Design review of the part built by this model. Coordinates are the model's own, in mm. Face numbers are marked on the shaded views. Coordinates: 2 decimals unless noted, no trailing zeros. Order: outer loops, then holes, each group sorted by start corner. A loop starts at its lowest first (then second) coordinate and runs counter-clockwise, first axis right, second up. Notation, with made-up numbers: (-37, 31.5) -> (6, 31.5) arc R24 ccw to (6, 50.5) -> close; hole circle Ø6 at (69.5, -5.75). An arc over 180 degrees is marked (long way). Use a Markdown table: item, result. Add a question column.
Q1. Add section C-C (y = 41). State the section outline as (x, z) points.
Q2. Add section D-D (x = 0). State the section outline as (y, z) points, then the cut area to 3 significant figures.
Q3. The part is to be moulded in two halves that separate along X. For the marked faces 1 and 2, say which applies: pulls with the +X half, pulls with the -X half, needs draft (parallel to the pull), parting line crosses it, or undercut.
Q4. Insertion check: pin 1 (0.5 mm diameter, centred on x = 1, z = 0, fed in from -Y); pin 2 (2 mm diameter, centred on x = -0.5, y = 3.5, fed in from +Z); pin 3 (2 mm diameter, centred on y = 7.5, z = -1.5, fed in from +X). Each pin has a flat end and moves straight along its axis. Give the tip position at first contact, or say it passes through.
Q5. Add section B-B (z = 0). State the section outline as (x, y) points.
Q6. Add section A-A (x = -2.2). State the section outline as (y, z) points.
Q7. Wall thickness on probe 1 along Y at (x, z) = (1.1, -1.85); probe 2 along Y at (x, z) = (-0.2, 0.3); probe 3 along Z at (x, y) = (1.05, 1): over which ranges is each line inside the solid? List them lowest first.
from build123d import *

# Parameters (mm, degrees)
F0_R     = 2.75
F1_DEPTH = 2
F3_DEPTH = 0.7
F4_R     = 1.5
F5_DEPTH = 45


with BuildPart() as f1:
    # F0 (on Front) → F1 (new body)
    with BuildSketch(Plane.XZ):
        Circle(F0_R)
    extrude(amount=F1_DEPTH)

    # F2 (on face) → F3 (cut)
    with BuildSketch(Plane.XZ.offset(2)):
        with BuildLine():
            ThreePointArc((2.75, 0), (2.7385168893, 0.2510482965), (2.7041634566, 0.5))
            Line((2.7041634566, 0.5), (-2.7041634566, 0.5))
            ThreePointArc((-2.7041634566, 0.5), (-2.75, 0), (-2.7041634566, -0.5))
            Line((-2.7041634566, -0.5), (2.7041634566, -0.5))
            ThreePointArc((2.7041634566, -0.5), (2.7385168893, -0.2510482965), (2.75, 0))
        make_face()
    extrude(amount=-F3_DEPTH, mode=Mode.SUBTRACT)

    # F4 (on face) → F5 (join)
    with BuildSketch(Plane(origin=(0, 0, 0), x_dir=(-1, 0, 0), z_dir=(0, 1, 0))):
        Circle(F4_R)
    extrude(amount=F5_DEPTH)


solid = f1.part
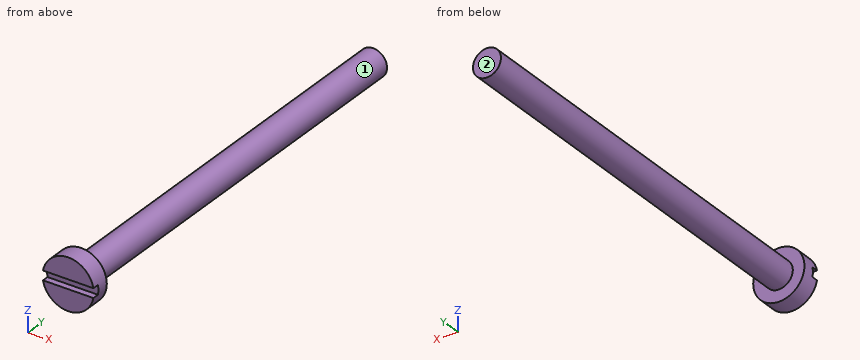
Established:
| question | item | result |
|---|---|---|
| 1 | outline | circle Ø3 at (0, 0) |
| 2 | outline | (-2, -2.75) -> (0, -2.75) -> (0, -1.5) -> (45, -1.5) -> (45, 1.5) -> (0, 1.5) -> (0, 2.75) -> (-2, 2.75) -> (-2, 0.5) -> (-1.3, 0.5) -> (-1.3, -0.5) -> (-2, -0.5) -> close |
| 2 | area | 145 mm^2 |
| 3 | face 1 | parting line crosses it |
| 3 | face 2 | needs draft |
| 4 | pin 1 | y = -1.3 |
| 4 | pin 2 | z = 1.5 |
| 4 | pin 3 | x = 1.41 |
| 5 | outline | (-2.75, -1.3) -> (2.75, -1.3) -> (2.75, 0) -> (1.5, 0) -> (1.5, 45) -> (-1.5, 45) -> (-1.5, 0) -> (-2.75, 0) -> close |
| 6 | outline | (-2, -1.65) -> (0, -1.65) -> (0, 1.65) -> (-2, 1.65) -> (-2, 0.5) -> (-1.3, 0.5) -> (-1.3, -0.5) -> (-2, -0.5) -> close |
| 7 | probe 1 | -2 to 0 |
| 7 | probe 2 | -1.3 to 45 |
| 7 | probe 3 | -1.07 to 1.07 |
